from build123d import *

# Parameters (mm, degrees)
SKETCH1_R                                        = 10
SKETCH1_R_2                                      = 1.1
BOSS_EXTRUDE1_DEPTH                              = 3.5
BOSS_EXTRUDE2_START                              = -3.5
BOSS_EXTRUDE2_DEPTH                              = 3.5
SKETCH8_R                                        = 16.129
BOSS_EXTRUDE4_DEPTH                              = 1.453
SKETCH9_W                                        = 26.35135
SKETCH9_H                                        = 1
CUT_EXTRUDE1_DEPTH                               = 23.2
CBORE_FOR_M2_HEX_HEAD_MACHINE_SCREW1_D           = 2.1
CBORE_FOR_M2_HEX_HEAD_MACHINE_SCREW1_DEPTH       = 3.5
CBORE_FOR_M2_HEX_HEAD_MACHINE_SCREW1_CBORE_D     = 4
CBORE_FOR_M2_HEX_HEAD_MACHINE_SCREW1_CBORE_DEPTH = 1.6
FILLET1_R                                        = 0.75
FILLET2_R                                        = 1


# Read off the part's stored shape, not the designer's step: Boss-Extrude2
with BuildPart() as part:
    # Sketch1 → Boss-Extrude1 (new body)
    with BuildSketch(Plane(origin=(0, 0, 0), x_dir=(1, 0, 0), z_dir=(0, 1, 0))):
        with BuildLine():
            Line((-18.5013, 8.509), (-18.5013, -8.491))
            Line((-18.5013, -8.491), (-15.0013, -16.862708425))
            ThreePointArc((-15.0013, -16.862708425), (0, -38.916709632), (15.0013, -16.862708425))
            Line((15.0013, -16.862708425), (18.4987, -8.491))
            Line((18.4987, -8.491), (18.4987, 8.509))
            ThreePointArc((18.4987, 8.509), (17.473573734, 10.983873734), (14.9987, 12.009))
            Line((14.9987, 12.009), (-15.0013, 12.009))
            ThreePointArc((-15.0013, 12.009), (-17.476173734, 10.983873734), (-18.5013, 8.509))
        make_face()
        with Locations(Location((0, -22.787709632, 0), (0, 0, 270))):
            Circle(SKETCH1_R, mode=Mode.SUBTRACT)
        with Locations(Location((-15.0013, 8.509, 0), (0, 0, 270))):
            Circle(SKETCH1_R_2, mode=Mode.SUBTRACT)
        with Locations(Location((-15.0013, -8.491, 0), (0, 0, 270))):
            Circle(SKETCH1_R_2, mode=Mode.SUBTRACT)
        with Locations(Location((14.9987, 8.509, 0), (0, 0, 270))):
            Circle(SKETCH1_R_2, mode=Mode.SUBTRACT)
        with Locations(Location((14.9987, -8.491, 0), (0, 0, 270))):
            Circle(SKETCH1_R_2, mode=Mode.SUBTRACT)
        Polygon((-11.95622235, -6.783455998), (11.95622235, -6.783455998), (11.95622235, -5.009), (15.0013, -5.009), (15.0013, 5.009), (11.95622235, 5.009), (11.95622235, 6.783455998), (9.9987, 6.783455998), (9.9987, 8.509), (-9.9987, 8.509), (-9.9987, 6.783455998), (-11.95622235, 6.783455998), (-11.95622235, 5.009), (-15.0013, 5.009), (-15.0013, -5.009), (-11.95622235, -5.009), align=None, mode=Mode.SUBTRACT)
    extrude(amount=BOSS_EXTRUDE1_DEPTH)

    # Boss-Extrude2 outline → Boss-Extrude2 (add)
    with BuildSketch(Plane(origin=(0, 3.5, 0), x_dir=(1, 0, 0), z_dir=(0, 1, 0)).offset(BOSS_EXTRUDE2_START)):
        with BuildLine():
            Line((-15.0013, -16.862708425), (-16.316803416, -13.716133844))
            ThreePointArc((-16.316803416, -13.716133844), (0.000574122, -41.456709624), (16.316245434, -13.71513029))
            Line((16.316245434, -13.71513029), (15.0013, -16.862708425))
            ThreePointArc((15.0013, -16.862708425), (0, -38.916709632), (-15.0013, -16.862708425))
        make_face()
        with BuildLine():
            Line((-9.612253982, -6.783455998), (9.612253982, -6.783455998))
            ThreePointArc((9.612253982, -6.783455998), (0, -4.118709632), (-9.612253982, -6.783455998))
        make_face()
    extrude(amount=BOSS_EXTRUDE2_DEPTH)

    # Sketch8 → Boss-Extrude4 (add)
    with BuildSketch(Plane(origin=(0, 3.5, 0), x_dir=(1, 0, 0), z_dir=(0, 1, 0))):
        with BuildLine():
            ThreePointArc((-16.316803416, -13.716133844), (-4.685784781, -40.859095356), (18.669, -22.787709632))
            ThreePointArc((18.669, -22.787709632), (18.071241615, -18.10136911), (16.316245434, -13.71513029))
            ThreePointArc((16.316245434, -13.71513029), (13.419530454, -9.808966882), (9.612253982, -6.783455998))
            ThreePointArc((9.612253982, -6.783455998), (0, -4.118709632), (-9.612253982, -6.783455998))
            ThreePointArc((-9.612253982, -6.783455998), (-13.419929579, -9.809379575), (-16.316803416, -13.716133844))
        make_face()
        with Locations(Location((0, -22.787709632, 0), (0, 0, 90))):
            Circle(SKETCH8_R, mode=Mode.SUBTRACT)
    extrude(amount=BOSS_EXTRUDE4_DEPTH)

    # Sketch9 → Cut-Extrude1 (cut)
    with BuildSketch(Plane(origin=(0, 0, -12.009), x_dir=(-1, 0, 0), z_dir=(0, 0, -1))):
        with Locations((0, 0.5)):
            Rectangle(SKETCH9_W, SKETCH9_H)
    extrude(amount=-CUT_EXTRUDE1_DEPTH, mode=Mode.SUBTRACT)

    # CBORE for M2 Hex Head Machine Screw1
    with Locations(Plane(origin=(0, 3.5, 0), x_dir=(1, 0, 0), z_dir=(0, 1, 0))):
        with Locations((-15.0013, 8.509), (14.9987, 8.509), (14.9987, -8.491), (-15.0013, -8.491)):
            CounterBoreHole(CBORE_FOR_M2_HEX_HEAD_MACHINE_SCREW1_D / 2, CBORE_FOR_M2_HEX_HEAD_MACHINE_SCREW1_CBORE_D / 2, CBORE_FOR_M2_HEX_HEAD_MACHINE_SCREW1_CBORE_DEPTH, depth=CBORE_FOR_M2_HEX_HEAD_MACHINE_SCREW1_DEPTH)

    # Fillet1
    fillet1_edges = [part.edges().sort_by_distance(p)[0] for p in [
        (9.9987, 2.25, -8.509),
        (-9.9987, 2.25, -8.509),
        (-9.9987, 2.25, -6.783455998),
        (-11.95622235, 2.25, -6.783455998),
        (-11.95622235, 2.25, -5.009),
        (-15.0013, 1.75, -5.009),
        (-15.0013, 1.75, 5.009),
        (-11.95622235, 2.25, 5.009),
        (-11.95622235, 2.25, 6.783455998),
        (11.95622235, 2.25, 6.783455998),
        (11.95622235, 2.25, 5.009),
        (15.0013, 1.75, 5.009),
        (15.0013, 1.75, -5.009),
        (11.95622235, 2.25, -5.009),
        (11.95622235, 2.25, -6.783455998),
        (9.9987, 2.25, -6.783455998),
    ]]
    fillet(fillet1_edges, radius=FILLET1_R)

    # Fillet2
    fillet2_edges = [part.edges().sort_by_distance(p)[0] for p in [
        (-18.669, 4.953, 22.787709632),
    ]]
    fillet(fillet2_edges, radius=FILLET2_R)


solid = part.part
The model under review builds one solid part; all positions refer to its coordinate system, in mm. A direction names the side the tool comes from. Round coordinates to 2 decimals unless told otherwise and drop trailing zeros. Write item = value, one per line. Start each with the question number.
Item 1: To check wall thickness, follow L1, parallel to Z at x = -0.5, y = 2.3; L2, parallel to X at y = 0.55, z = 22.5; L3, parallel to Z at x = 0.5, y = 3.65. State the ranges of each line that lie inside material, in increasing order.
Item 2: For faces 1 (the flat face through (-13.176, 0.5, 8.1)), 2 (the flat face through (13, 2, -5.009)), 3 (the cylindrical face through (9.8, 4.2, 35.6)), list the 3-axis set-ups (+Z, -Z, +X, -X, +Y, -Y) from which the entire face can be reached by the end or side of a thin tool; tool diameter is ignored.
Item 3: Mouldability with a two-part tool opening along X and no side actions: class faces 4 (the flat face through (17.39, 1.73, 11.14)), 5 (the flat face through (8, 0, 14)), 6 (the flat face through (0.2, 0.5, 11.191)) as released by +X, released by -X, zero draft, split by the parting line, or undercut.
Item 4: Insertion check: pin 1 (1.8 mm diameter, centred on x = 15, z = 8.49, fed in from +Y); pin 2 (4.5 mm diameter, centred on x = -15, z = -8.5, fed in from +Y); pin 3 (1.7 mm diameter, centred on x = -13.5, y = 2, fed in from +Z); pin 4 (1.2 mm diameter, centred on x = 15.5, z = -9, fed in from +Y). Each pin has a flat end and moves straight along its axis. Give the tip position at first contact, or say it passes through.
Item 5: Take a section at A-A on x = 0. Count the separate pieces of the cut face and the enclosed holes in it, plus the area to 3 significant figures.
Result:
q1.L1 = -12.01 to -8.51, 4.13 to 12.8, 32.78 to 41.45
q1.L2 = -18.67 to -10, 10 to 18.67
q1.L3 = 4.13 to 6.67, 38.91 to 41.45
q2.face_1 = -Z, -Y
q2.face_2 = +Y, -Y
q2.face_3 = +Y
q3.face_4 = released by +X
q3.face_5 = zero draft
q3.face_6 = undercut
q4.pin_1 = through
q4.pin_2 = 3.5
q4.pin_3 = 36.52
q4.pin_4 = 1.9
q5.separate_pieces = 3
q5.enclosed_holes = 0
q5.area = 69.3 mm²
